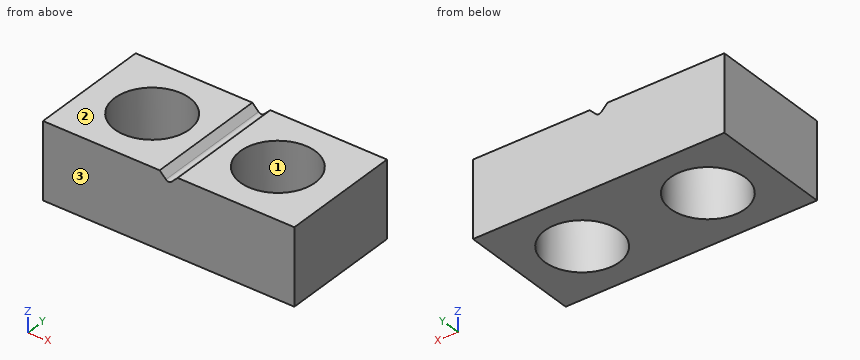
```python
from build123d import *

# Parameters (mm, degrees)
SKETCH2_W               = 16.51
SKETCH2_H               = 8
SKETCH2_R               = 2.45745
BASE_EXTRUDE_DEPTH      = 5
CUT_EXTRUDE2_DEPTH      = 5
CUT_EXTRUDE2_DEPTH_BACK = 5


with BuildPart() as part:
    # Sketch2 → Base-Extrude (new body)
    with BuildSketch(Plane.XY):
        Rectangle(SKETCH2_W, SKETCH2_H)
        with Locations((4.1275, 0)):
            Circle(SKETCH2_R, mode=Mode.SUBTRACT)
        with Locations(Location((-4.1275, 0, 0), (0, 0, 180))):  # turned: the seam where the file's is
            Circle(SKETCH2_R, mode=Mode.SUBTRACT)
    extrude(amount=-BASE_EXTRUDE_DEPTH)

    # Sketch3 → Cut-Extrude2 (cut, two sides)
    with BuildSketch(Plane(origin=(0, 0, 0), x_dir=(-1, 0, 0), z_dir=(0, 1, 0))) as cut_extrude2_sk:
        with BuildLine():
            Line((0.590493938, 0), (0.179605122, -0.410888816))
            ThreePointArc((0.179605122, -0.410888816), (0, -0.485283694), (-0.179605122, -0.410888816))
            Line((-0.179605122, -0.410888816), (-0.590493938, 0))
            Line((-0.590493938, 0), (0.590493938, 0))
        make_face()
    extrude(amount=CUT_EXTRUDE2_DEPTH, mode=Mode.SUBTRACT)
    extrude(cut_extrude2_sk.sketch, amount=-CUT_EXTRUDE2_DEPTH_BACK, mode=Mode.SUBTRACT)


solid = part.part
```
CAD build for the part. Positions are in the model's coordinates, mm. Face numbers are marked on the shaded views. Give positions to 0.01 mm unless a question says otherwise; leave off trailing zeros. Loops run counter-clockwise (first coordinate to the right, second up) from the corner with the lowest first, then second, coordinate; pieces in that order, holes last. Notation, with made-up numbers: M 9,-4.75 L 48,-4.75 A34 ccw 48,32.25 Z; hole C 71.25,41 d6. An arc over 180 degrees is marked long. Use one line per item in the form item = value.
Item 1: Drill centre lines: probe 1 along X at (y, z) = (0.25, -0.7) (3 decimals); probe 2 along X at (y, z) = (2, -3.8) (3 decimals); probe 3 along Y at (x, z) = (-3.75, -0.15). Where is each one in solid material? Low to high. Write a range as from..to.
Determined:
probe_1 = -8.255..-6.572, -1.683..1.683, 6.572..8.255
probe_2 = -8.255..-5.555, -2.7..2.7, 5.555..8.255
probe_3 = -4..-2.43, 2.43..4
Item 2: Two-plate mould, pull along Y, no slides. Class the marked faces 1, 2 and 3: pulls with the +Y half, pulls with the -Y half, needs draft (parallel to the pull), parting line crosses it, or undercut.
Determined:
face_1 = undercut
face_2 = needs draft
face_3 = pulls with the -Y half
Item 3: Slice it at B-B (x = -5.5). List the corners of the cut face in (y, z), plus the area to 3 significant figures.
Determined:
outline = M -4,-5 L -2.04,-5 L -2.04,0 L -4,0 Z; M 2.04,-5 L 4,-5 L 4,0 L 2.04,0 Z
area = 19.6 mm2
Item 4: Slice it at A-A (y = 0). Count the separate pieces of the cut face and the enclosed holes in it, plus the area to 3 significant figures.
Determined:
separate_pieces = 3
enclosed_holes = 0
area = 33.1 mm2
Item 5: Slice it at C-C (z = -2.75). List the corners of the cut face in (x, y) (1 decimal), plus the area to 3 significant figures.
Determined:
outline = M -8.3,-4 L 8.3,-4 L 8.3,4 L -8.3,4 Z; hole C -4.1,0 d4.9; hole C 4.1,0 d4.9
area = 94.1 mm2
